from build123d import *

# Parameters (mm, degrees)
F0_R     = 10.16
F1_DEPTH = 15.7734
F2_DEPTH = 40.2336
F3_SIZE  = 3.302


# Not quite as in the source:
# - a feature names something its author has since deleted; it is built from what else it names


with BuildPart() as f1:
    # F0 (on Top) → F1 (new body)
    with BuildSketch(Plane.XY):
        with BuildLine():
            ThreePointArc((5.2429423077, 28.0898946413), (21.9812158608, 18.258060529), (28.575, 0))
            ThreePointArc((28.575, 0), (21.9291125509, -18.3206071879), (5.0828111824, -28.1193110777))
            Line((5.0828111824, -28.1193110777), (55.6786843639, -18.9736648961))
            ThreePointArc((55.6786843639, -18.9736648961), (34.9510761924, -0.9964050199), (53.687254757, 19.0478267179))
            Line((53.687254757, 19.0478267179), (5.2429423077, 28.0898946413))
        make_face()
        with BuildLine():
            ThreePointArc((73.025, 0), (67.3432637826, 13.5717361984), (53.687254757, 19.0478267179))
            ThreePointArc((53.687254757, 19.0478267179), (34.9510761924, -0.9964050199), (55.6786843639, -18.9736648961))
            ThreePointArc((55.6786843639, -18.9736648961), (68.0348308513, -12.8539354454), (73.025, 0))
        make_face()
        with Locations((53.975, 0)):
            Circle(F0_R, mode=Mode.SUBTRACT)
    extrude(amount=F1_DEPTH)

    # F0 (on Top) → F2 (join)
    with BuildSketch(Plane.XY):
        with BuildLine():
            ThreePointArc((5.0828111824, -28.1193110777), (21.9291125509, -18.3206071879), (28.575, 0))
            ThreePointArc((28.575, 0), (21.9812158608, 18.258060529), (5.2429423077, 28.0898946413))
            ThreePointArc((5.2429423077, 28.0898946413), (-28.5748840448, 0.0814053193), (5.0828111824, -28.1193110777))
        make_face()
        with BuildLine():
            ThreePointArc((13.4477648793, -4.826), (-14.2875, 0), (13.4477648793, 4.826))
            Line((13.4477648793, 4.826), (18.5293, 4.826))
            Line((18.5293, 4.826), (18.5293, 0))
            Line((18.5293, 0), (18.5293, -4.826))
            Line((18.5293, -4.826), (13.4477648793, -4.826))
        make_face(mode=Mode.SUBTRACT)
    extrude(amount=F2_DEPTH)

    # F3
    f3_edges = [f1.edges().sort_by_distance(p)[0] for p in [
        (-5.082811, 28.119311, 40.2336),
    ]]
    chamfer(f3_edges, length=F3_SIZE)


solid = f1.part
Model file for the job. Use its own axes, mm. A direction names the side the tool comes from. Round coordinates to 2 decimals unless told otherwise and drop trailing zeros. Loops run counter-clockwise (first coordinate to the right, second up) from the corner with the lowest first, then second, coordinate; pieces in that order, holes last. Notation, with made-up numbers: (55, 15) - (108, 15) arc R36 ccw to (108, 52) - close; hole circle Ø6 at (-30, 34.5). An arc over 180 degrees is marked (long way). Write each question's results on one line, items separated by ' | '.
(1) Saw through at D-D, the plane x = 50.5. List the corners of the cut face in (y, z).
Answer below:
outline: (-19.91, 0) - (-9.55, 0) - (-9.55, 15.77) - (-19.91, 15.77) - close; (9.55, 0) - (19.64, 0) - (19.64, 15.77) - (9.55, 15.77) - close
(2) Saw through at A-A, the plane x = 0. List the corners of the cut face in (y, z) (1 decimal), then the cut area to 3 significant figures.
Answer below:
outline: (-28.6, 0) - (-14.3, 0) - (-14.3, 40.2) - (-25.3, 40.2) - (-28.6, 36.9) - close; (14.3, 0) - (28.6, 0) - (28.6, 36.9) - (25.3, 40.2) - (14.3, 40.2) - close | area: 1,140 mm^2
(3) Saw through at C-C, the plane z = 13.5. Count the separate pieces of the cut face and the enclosed holes in it, then the cut area to 3 significant figures.
Answer below:
separate pieces: 1 | enclosed holes: 2 | area: 3,440 mm^2
(4) Pin check, flat tips, straight feed: pin 1 (12 mm diameter, centred on x = 53.975, y = 0, fed in from -Z); pin 2 (5.5 mm diameter, centred on x = 15.5, z = 13, fed in from +Y); pin 3 (6 mm diameter, centred on x = 52, z = 7.5, fed in from -Y); pin 4 (1 mm diameter, centred on x = -13.5, y = -12, fed in from -Z). Stop position of each tip, or through.
Answer below:
pin 1: passes through | pin 2: stops at y = 26.69 | pin 3: stops at y = -20.18 | pin 4: stops at z = 0
(5) Wall check: L1, parallel to Y at x = 0, z = 18 (1 decimal); L2, parallel to X at y = 6, z = 13.5; L3, parallel to Z at x = 32.5, y = 1. Give the ranges that are in metal, low to high.
Answer below:
L1: y = -28.6 to -14.3, 14.3 to 28.6 | L2: x = -27.94 to -12.97, 12.97 to 45.78, 62.17 to 72.06 | L3: z = 0 to 15.77
(6) 3-axis set-ups, long thin cutter, end or side, ignore diameter. For faces 4 (the flat face through (18.529, 0, 20)), 5 (the flat face through (30.03, -23.61, 7.78)): which of +Z, -Z, +X, -X, +Y, -Y reach the whole face in a straight line?
Answer below:
face 4: +Z, -Z | face 5: +Z, -Z, +X, -Y
(7) Mould opens along Y. For faces 1 (the flat face through (29.804, 23.506, 7.776)), 2 (the cylindrical face through (-14.277, -0.559, 19.835)), 3 (the flat face through (22, 0, 0)) say: released by +Y, released by -Y, zero draft, split by the parting line, or undercut.
Answer below:
face 1: released by +Y | face 2: undercut | face 3: zero draft
